```python
from build123d import *

# Parameters (mm, degrees)
F2_T     = -2.5
F3_DEPTH = 10
F4_R     = 5
F5_R     = 1
F6_R     = 3


with BuildPart() as f1:
    # F0 (on Front) → F1 (revolve)
    with BuildSketch(Plane.XZ):
        Polygon((0, 44.5134416223), (-35.1207107306, 44.5134416223), (-26.3405442238, 0), (0, 0), align=None)
    revolve(axis=Axis((0, 0, 22.2567208111), (0, 0, 1)))

    # F2
    f2_openings = [f1.faces().sort_by_distance(p)[0] for p in [
        (0, 0, 44.513442),
    ]]
    offset(amount=F2_T, openings=f2_openings)

    # F3 (add): a face of the model
    f3_faces = [f1.faces().sort_by_distance(p)[0] for p in [
        (0, 0, 0),
    ]]
    extrude(f3_faces, amount=F3_DEPTH)

    # F4
    f4_edges = [f1.edges().sort_by_distance(p)[0] for p in [
        (24.285494, 0, 2.5),
    ]]
    fillet(f4_edges, radius=F4_R)

    # F5
    f5_edges = [f1.edges().sort_by_distance(p)[0] for p in [
        (32.572542, 0, 44.513442),
        (35.120711, 0, 44.513442),
    ]]
    fillet(f5_edges, radius=F5_R)

    # F6
    f6_edges = [f1.edges().sort_by_distance(p)[0] for p in [
        (26.340544, 0, -10),
    ]]
    fillet(f6_edges, radius=F6_R)


solid = f1.part
```
Check sheet for the modelled part. Datum: model origin and axes. Units: mm. Round coordinates to 2 decimals unless told otherwise and drop trailing zeros. Loops run counter-clockwise (first coordinate to the right, second up) from the corner with the lowest first, then second, coordinate; pieces in that order, holes last. Notation, with made-up numbers: (-3.75, -18.75) - (6.25, -18.75) arc R26 ccw to (6.25, 6.25) - close; hole circle Ø8 at (-2.5, 78.25). An arc over 180 degrees is marked (long way). Answer as a JSON object with one key per item and string values. Group by question number.
Q1. Scan lines: line 1 along Z through (x, y) = (7, 16.5); line 2 along Y through (x, z) = (-24.5, 23); line 3 along X through (y, z) = (2.5, 22). Record each from-to range of solid material in increasing order. Write a range as [from, to].
Q2. Mould release check, pull along X, two halves, no side actions. Record for faces 1 (the face through (0, 0, -10)), 2 (the face through (-25.124, -7.912, -3.451)), 3 (the face through (0, 0, 2.5)): released by +X, released by -X, zero draft, split by the parting line, or undercut.
Q3. Sectioned sample at C-C, the plane z = 34. Enter the section's corners in (x, y).
Q4. Sectioned sample at D-D, the plane z = 8. Enter the section's corners in (x, y).
Q5. Sectioned sample at A-A, the plane x = 0. Enter the section's corners in (y, z).
Q6. Gauge pin test, flat ends, axial feed: P1, Ø1.5, axis at y = 24, z = -3, coming from the +X side; P2, Ø1, axis at x = -18.5, z = 2, coming from the -Y side; P3, Ø8, axis at y = -5, z = 6.5, coming from the +X side. Record the tip position at first contact, or that the pin passes through.
Solution:
{
 "1": {"line 1": "z = [-10, 2.5]", "line 2": "y = [-18.79, -14.22], [14.22, 18.79]", "line 3": "x = [-30.58, -28.02], [28.02, 30.58]"},
 "2": {"face 1": "zero draft", "face 2": "split by the parting line", "face 3": "undercut"},
 "3": {"outline": "circle Ø66.09 at (0, 0); hole circle Ø61 at (0, 0)"},
 "4": {"outline": "circle Ø55.84 at (0, 0); hole circle Ø50.74 at (0, 0)"},
 "5": {"outline": "(-34.89, 43.32) - (-26.34, 0) - (-26.34, -7) arc R3 ccw to (-23.34, -10) - (23.34, -10) arc R3 ccw to (26.34, -7) - (26.34, 0) - (34.89, 43.32) arc R1 ccw to (33.9, 44.51) - (33.39, 44.51) arc R1 ccw to (32.41, 43.71) - (25.08, 6.53) arc R5 cw to (20.18, 2.5) - (-20.18, 2.5) arc R5 cw to (-25.08, 6.53) - (-32.41, 43.71) arc R1 ccw to (-33.39, 44.51) - (-33.9, 44.51) arc R1 ccw to start"},
 "6": {"P1": "stops at x = 12.38", "P2": "stops at y = -19.79", "P3": "stops at x = 28.15"}
}
